CAD build for the part. Positions are in the model's coordinates, mm. A direction names the side the tool comes from. Round coordinates to 2 decimals unless told otherwise and drop trailing zeros. Order: outer loops, then holes, each group sorted by start corner. A loop starts at its lowest first (then second) coordinate and runs counter-clockwise, first axis right, second up. Notation, with made-up numbers: (-5, 57) -> (48, 57) arc R18 ccw to (48, 79) -> close; hole circle Ø3 at (45.25, 84). An arc over 180 degrees is marked (long way). Answer as CSV lines item,"result". Start each with the question number.
from build123d import *

# Parameters (mm, degrees)
ESBO_O1_W                     = 18
ESBO_O1_H                     = 23.7
RESSALTO_EXTRUS_O1_DEPTH      = 1.1
RESSALTO_EXTRUS_O2_DEPTH      = 1.1
RESSALTO_EXTRUS_O2_DEPTH_BACK = 5.6


with BuildPart() as part:
    # Esboço1 → Ressalto-extrusão1 (new body)
    with BuildSketch(Plane(origin=(0, 0, 0), x_dir=(1, 0, 0), z_dir=(0, 1, 0))):
        with Locations((9, 11.85)):
            Rectangle(ESBO_O1_W, ESBO_O1_H)
    extrude(amount=RESSALTO_EXTRUS_O1_DEPTH)

    # Esboço2 → Ressalto-extrusão2 (add, two sides)
    with BuildSketch(Plane.ZY) as ressalto_extrus_o2_sk:
        with BuildLine():
            Line((-8.7, 4.1), (-3, 4.1))
            ThreePointArc((-3, 4.1), (-1.5, 2.6), (-3, 1.1))
            Line((-3, 1.1), (-8.7, 1.1))
            ThreePointArc((-8.7, 1.1), (-10.2, 2.6), (-8.7, 4.1))
        make_face()
    extrude(amount=RESSALTO_EXTRUS_O2_DEPTH)
    extrude(ressalto_extrus_o2_sk.sketch, amount=-RESSALTO_EXTRUS_O2_DEPTH_BACK)


solid = part.part
Item 1: Band-saw the part on C-C, the plane y = 2.6. Give the cut face in (x, z).
Item 2: Pin check, flat tips, straight feed: pin 1 (10 mm diameter, centred on x = 12.5, z = -10, fed in from +Y); pin 2 (0.9 mm diameter, centred on x = -0.5, z = -6.5, fed in from -Y); pin 3 (2 mm diameter, centred on x = 5.5, y = 2.5, fed in from -Z). Stop position of each tip, or through.
Item 3: Band-saw the part on A-A, the plane x = 2.25. Give the cut face in (y, z), and give its area (3 significant figures).
Item 4: Mould opens along Y. For faces 1 (the flat face through (8.9, 0.5, 0)), 2 (the cylindrical face through (2.2, 2.6, -1.5)), 3 (the flat face through (2, 4.1, -6)) say: released by +Y, released by -Y, zero draft, split by the parting line, or undercut.
Item 5: Tool access for faces 4 (the flat face through (5.6, 3, -6)), 5 (the flat face through (0, 0.5, -11.7)), 6 (the flat face through (-1.1, 3, -6)): list every direction of +Z, -Z, +X, -X, +Y, -Y with a clear straight run to the whole face (end or side of a thin tool).
Item 6: Band-saw the part on D-D, the plane x = 13.75. Give the cut face in (y, z).
Item 7: Probe line 1 (Y direction, x = 6, z = -2.25); line 2 (X direction, y = 0.3, z = -4.5); line 3 (X direction, y = 2.6, z = -7). List the from-to ranges inside material, lowest first.
Item 8: Band-saw the part on B-B, the plane z = -6. Give the cut face in (x, y), and give its area (3 significant figures).
Values:
1,outline,"(-1.1, -10.2) -> (5.6, -10.2) -> (5.6, -1.5) -> (-1.1, -1.5) -> close"
2,pin 1,"y = 1.1"
2,pin 2,"y = 1.1"
2,pin 3,"z = -10.2"
3,outline,"(0, -23.7) -> (1.1, -23.7) -> (1.1, -8.7) arc R1.5 ccw to (4.1, -8.7) -> (4.1, -3) arc R1.5 ccw to (1.1, -3) -> (1.1, 0) -> (0, 0) -> close"
3,area,"50.2 mm²"
4,face 1,"zero draft"
4,face 2,"undercut"
4,face 3,"released by +Y"
5,face 4,"+Z, -Z, +X, +Y"
5,face 5,"+Z, -Z, -X, -Y"
5,face 6,"+Z, -Z, -X, +Y, -Y"
6,outline,"(0, -23.7) -> (1.1, -23.7) -> (1.1, 0) -> (0, 0) -> close"
7,line 1,"0 to 1.1"
7,line 2,"0 to 18"
7,line 3,"-1.1 to 5.6"
8,outline,"(-1.1, 1.1) -> (0, 1.1) -> (0, 0) -> (18, 0) -> (18, 1.1) -> (5.6, 1.1) -> (5.6, 4.1) -> (-1.1, 4.1) -> close"
8,area,"39.9 mm²"
